CAD build for the part. Positions are in the model's coordinates, mm. Coordinates: 2 decimals unless noted, no trailing zeros. Answer as a JSON object with one key per item and string values. Group by question number.
from build123d import *

# Parameters (mm, degrees)
PAD_DEPTH       = 400
SKETCH001_R     = 3.25
POCKET_DEPTH    = 21
SKETCH002_R     = 5.5
POCKET001_DEPTH = 2


with BuildPart() as part:
    # Sketch → Pad (new body)
    with BuildSketch(Plane.YZ):
        with BuildLine():
            Line((0, 4.1), (0.65, 4.5))
            Line((0.65, 4.5), (3, 4.5))
            Line((3, 4.5), (5.5, 7))
            Line((5.5, 7), (5.5, 8.5))
            Line((5.5, 8.5), (3, 8.5))
            Line((3, 8.5), (3, 9.5))
            Line((3, 9.5), (3.5, 9.5))
            Line((3.5, 9.5), (3.5, 10))
            Line((3.5, 10), (8.5, 10))
            ThreePointArc((10, 8.5), (9.56066, 9.56066), (8.5, 10))
            Line((10, 8.5), (10, 3.5))
            Line((10, 3.5), (9.5, 3.5))
            Line((9.5, 3.5), (9.5, 3))
            Line((9.5, 3), (8.5, 3))
            Line((8.5, 3), (8.5, 5.5))
            Line((8.5, 5.5), (7, 5.5))
            Line((7, 5.5), (4.5, 3))
            Line((4.5, 3), (4.5, 0.65))
            Line((4.5, 0.65), (4.1, 0))
            Line((4.5, -0.65), (4.1, 0))
            Line((4.5, -3), (4.5, -0.65))
            Line((7, -5.5), (4.5, -3))
            Line((8.5, -5.5), (7, -5.5))
            Line((8.5, -3), (8.5, -5.5))
            Line((9.5, -3), (8.5, -3))
            Line((9.5, -3.5), (9.5, -3))
            Line((10, -3.5), (9.5, -3.5))
            Line((10, -8.5), (10, -3.5))
            ThreePointArc((8.5, -10), (9.56066, -9.56066), (10, -8.5))
            Line((3.5, -10), (8.5, -10))
            Line((3.5, -9.5), (3.5, -10))
            Line((3, -9.5), (3.5, -9.5))
            Line((3, -8.5), (3, -9.5))
            Line((5.5, -8.5), (3, -8.5))
            Line((5.5, -7), (5.5, -8.5))
            Line((3, -4.5), (5.5, -7))
            Line((0.65, -4.5), (3, -4.5))
            Line((0, -4.1), (0.65, -4.5))
            Line((0, -4.1), (-0.65, -4.5))
            Line((-0.65, -4.5), (-3, -4.5))
            Line((-3, -4.5), (-5.5, -7))
            Line((-5.5, -7), (-5.5, -8.5))
            Line((-5.5, -8.5), (-3, -8.5))
            Line((-3, -8.5), (-3, -9.5))
            Line((-3, -9.5), (-3.5, -9.5))
            Line((-3.5, -9.5), (-3.5, -10))
            Line((-3.5, -10), (-8.5, -10))
            ThreePointArc((-10, -8.5), (-9.56066, -9.56066), (-8.5, -10))
            Line((-10, -8.5), (-10, -3.5))
            Line((-10, -3.5), (-9.5, -3.5))
            Line((-9.5, -3.5), (-9.5, -3))
            Line((-9.5, -3), (-8.5, -3))
            Line((-8.5, -3), (-8.5, -5.5))
            Line((-8.5, -5.5), (-7, -5.5))
            Line((-7, -5.5), (-4.5, -3))
            Line((-4.5, -3), (-4.5, -0.65))
            Line((-4.5, -0.65), (-4.1, 0))
            Line((-4.5, 0.65), (-4.1, 0))
            Line((-4.5, 3), (-4.5, 0.65))
            Line((-7, 5.5), (-4.5, 3))
            Line((-8.5, 5.5), (-7, 5.5))
            Line((-8.5, 3), (-8.5, 5.5))
            Line((-9.5, 3), (-8.5, 3))
            Line((-9.5, 3.5), (-9.5, 3))
            Line((-10, 3.5), (-9.5, 3.5))
            Line((-10, 8.5), (-10, 3.5))
            ThreePointArc((-8.5, 10), (-9.56066, 9.56066), (-10, 8.5))
            Line((-3.5, 10), (-8.5, 10))
            Line((-3.5, 9.5), (-3.5, 10))
            Line((-3, 9.5), (-3.5, 9.5))
            Line((-3, 8.5), (-3, 9.5))
            Line((-5.5, 8.5), (-3, 8.5))
            Line((-5.5, 7), (-5.5, 8.5))
            Line((-3, 4.5), (-5.5, 7))
            Line((-0.65, 4.5), (-3, 4.5))
            Line((0, 4.1), (-0.65, 4.5))
        make_face()
        with BuildLine():
            Line((1.340499, 2.401159), (1.923239, 2.983899))
            Line((1.923239, 2.983899), (2.983899, 1.923239))
            Line((2.983899, 1.923239), (2.401159, 1.340499))
            ThreePointArc((2.75, 0), (2.661361, 0.692573), (2.401159, 1.340499))
            ThreePointArc((2.401164, -1.34049), (2.661362, -0.692568), (2.75, 0))
            Line((2.983904, -1.92323), (2.401164, -1.34049))
            Line((1.923247, -2.983894), (2.983904, -1.92323))
            Line((1.340507, -2.401154), (1.923247, -2.983894))
            ThreePointArc((0, -2.75), (0.692577, -2.66136), (1.340507, -2.401154))
            ThreePointArc((-1.340507, -2.401154), (-0.692577, -2.66136), (0, -2.75))
            Line((-1.340507, -2.401154), (-1.923247, -2.983894))
            Line((-1.923247, -2.983894), (-2.983904, -1.92323))
            Line((-2.983904, -1.92323), (-2.401164, -1.34049))
            ThreePointArc((-2.75, 0), (-2.661362, -0.692568), (-2.401164, -1.34049))
            ThreePointArc((-2.401159, 1.340499), (-2.661361, 0.692572), (-2.75, 0))
            Line((-2.983899, 1.923239), (-2.401159, 1.340499))
            Line((-1.923239, 2.983899), (-2.983899, 1.923239))
            Line((-1.340499, 2.401159), (-1.923239, 2.983899))
            ThreePointArc((0, 2.75), (-0.692573, 2.661361), (-1.340499, 2.401159))
            ThreePointArc((1.340499, 2.401159), (0.692573, 2.661361), (0, 2.75))
        make_face(mode=Mode.SUBTRACT)
    extrude(amount=PAD_DEPTH)

    # Sketch001 → Pocket (cut)
    with BuildSketch(Plane.XY.offset(10)):
        with Locations((165, 0)):
            Circle(SKETCH001_R)
    extrude(amount=-POCKET_DEPTH, mode=Mode.SUBTRACT)

    # Sketch002 → Pocket001 (cut)
    with BuildSketch(Plane.XY.offset(10)):
        with Locations((165, 0)):
            Circle(SKETCH002_R)
    extrude(amount=-POCKET001_DEPTH, mode=Mode.SUBTRACT)


solid = part.part
Item 1: Flat gauge pins, fed straight in: P1, Ø12, axis at y = 7, z = 3.5, coming from the +X side; P2, Ø0.5, axis at x = 230.5, z = -9, coming from the -Y side; P3, Ø0.6, axis at x = 300, z = 9.5, coming from the +Y side; P4, Ø0.8, axis at x = 41.5, z = 9, coming from the +Y side. Where does each tip first touch, or does it go through?
Item 2: Drill centre lines: L1, parallel to Y at x = 97, z = 3.25; L2, parallel to Y at x = 351.5, z = 7.5; L3, parallel to X at y = -2.75, z = 4.25. Where is each one in solid material? Low to high.
Item 3: Pull direction Y, two halves, no side cores. Call faces 1 (the cylindrical face through (166.5, -2.883, 0.067)), 2 (the flat face through (0, -2, -4)): +Y half, -Y half, draft (parallel to the pull), parting line (faces both ways), or undercut.
Reply:
{
 "1": {"P1": "x = 400", "P2": "y = -9.98", "P3": "y = 9.83", "P4": "y = 10"},
 "2": {"L1": "-9.5 to -8.5, -4.75 to 4.75, 8.5 to 9.5", "L2": "-10 to -5.5, 5.5 to 10", "L3": "0 to 163.27, 166.73 to 400"},
 "3": {"face 1": "undercut", "face 2": "draft"}
}
